```python
from build123d import *

# Parameters (mm, degrees)
SKETCH1_R           = 11
SKETCH1_R_2         = 4
SKETCH1_R_3         = 1.7
BOSS_EXTRUDE1_DEPTH = 3.5
SKETCH2_R           = 5
BOSS_EXTRUDE2_DEPTH = 10
SKETCH2_2_R         = 5
BOSS_EXTRUDE3_DEPTH = 5
SKETCH3_R           = 4
CUT_EXTRUDE1_DEPTH  = 20


with BuildPart() as part:
    # Sketch1 → Boss-Extrude1 (new body)
    with BuildSketch(Plane(origin=(0, 0, 0), x_dir=(1, 0, 0), z_dir=(0, 1, 0))):
        with Locations((-13.832754598, -13.4034603)):
            Circle(SKETCH1_R)
        with Locations((-13.832754598, -13.4034603)):
            Circle(SKETCH1_R_2, mode=Mode.SUBTRACT)
        with Locations((-19.382754598, -7.8534603)):
            Circle(SKETCH1_R_3, mode=Mode.SUBTRACT)
        with Locations((-8.282754598, -7.8534603)):
            Circle(SKETCH1_R_3, mode=Mode.SUBTRACT)
        with Locations((-8.282754598, -18.9534603)):
            Circle(SKETCH1_R_3, mode=Mode.SUBTRACT)
        with Locations((-19.382754598, -18.9534603)):
            Circle(SKETCH1_R_3, mode=Mode.SUBTRACT)
    extrude(amount=BOSS_EXTRUDE1_DEPTH)

    # Sketch2 → Boss-Extrude2 (add)
    with BuildSketch(Plane(origin=(0, 3.5, 0), x_dir=(1, 0, 0), z_dir=(0, 1, 0))):
        with Locations((-13.832754598, -13.4034603)):
            Circle(SKETCH2_R)
    extrude(amount=BOSS_EXTRUDE2_DEPTH)

    # Sketch2_2 → Boss-Extrude3 (add)
    with BuildSketch(Plane(origin=(0, 3.5, 0), x_dir=(1, 0, 0), z_dir=(0, 1, 0))):
        with Locations((-13.832754598, -13.4034603)):
            Circle(SKETCH2_2_R)
    extrude(amount=-BOSS_EXTRUDE3_DEPTH)

    # Sketch3 → Cut-Extrude1 (cut)
    with BuildSketch(Plane(origin=(0, 13.5, 0), x_dir=(1, 0, 0), z_dir=(0, 1, 0))):
        with Locations((-13.832754598, -13.4034603)):
            Circle(SKETCH3_R)
    extrude(amount=-CUT_EXTRUDE1_DEPTH, mode=Mode.SUBTRACT)


solid = part.part
```
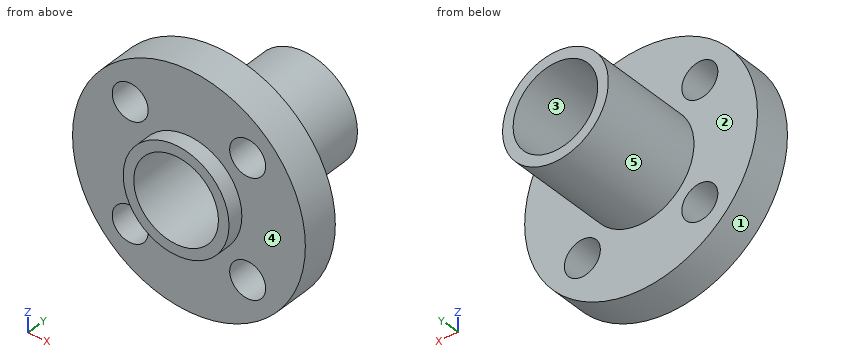
Design review of the part built by this model. Coordinates are the model's own, in mm. Face numbers are marked on the shaded views. A direction names the side the tool comes from. Give positions to 0.01 mm unless a question says otherwise; leave off trailing zeros. Loops run counter-clockwise (first coordinate to the right, second up) from the corner with the lowest first, then second, coordinate; pieces in that order, holes last. Notation, with made-up numbers: M 75,-23 L 110,-23 A12 ccw 110,-3 Z; hole C 61.5,52 d3. An arc over 180 degrees is marked long. Return JSON: item names as keys, results as strings. Group by question number.
Item 1: We need section A-A (z = 7.5). Give the boundary of the cut face in (x, y), and give its area (3 significant figures).
Item 2: Insertion check: pin 1 Ø1.5 at (y, z) = (6.5, 16) entering from -X; pin 2 Ø4.5 at (x, z) = (-8.28, 7.85) entering from -Y; pin 3 Ø8 at (y, z) = (6, 18.5) entering from -X. Each pin has a flat end and moves straight along its axis. Give the tip position at first contact, or say it passes through.
Item 3: Tool access review of the marked faces 1 and 2: name each direction out of +Z, -Z, +X, -X, +Y, -Y from which nothing blocks a thin tool from reaching the whole face with its end or side.
Item 4: Mouldability with a two-part tool opening along X and no side actions: class the marked faces 3, 4 and 5 as released by +X, released by -X, zero draft, split by the parting line, or undercut.
Item 5: We need section B-B (x = -16.5). Give the boundary of the cut face in (y, z).
Item 6: For probe 1 along Z at (x, y) = (-8.25, 0.5); probe 2 along Y at (x, z) = (-12, 18.25); probe 3 along Z at (x, y) = (-6.75, 0.25), list the stretches that pass through material, from the lowest coordinate up.
Item 7: We need section D-D (x = -8). Give the boundary of the cut face in (y, z).
Item 8: We need section C-C (z = 16). Give the boundary of the cut face in (x, y), and give its area (3 significant figures).
Output:
{
 "1": {"outline": "M -23.11,0 L -21.05,0 L -21.05,3.5 L -23.11,3.5 Z; M -17.72,0 L -9.95,0 L -9.95,3.5 L -17.72,3.5 Z; M -6.62,0 L -4.55,0 L -4.55,3.5 L -6.62,3.5 Z", "area": "41.7 mm^2"},
 "2": {"pin 1": "stops at x = -18.48", "pin 2": "stops at y = 0", "pin 3": "stops at x = -24.65"},
 "3": {"face 1": "+Y, -Y", "face 2": "+Y"},
 "4": {"face 3": "undercut", "face 4": "zero draft", "face 5": "split by the parting line"},
 "5": {"outline": "M -1.5,9.17 L 0,9.17 L 0,2.73 L 3.5,2.73 L 3.5,9.17 L 13.5,9.17 L 13.5,10.42 L -1.5,10.42 Z; M -1.5,16.38 L 13.5,16.38 L 13.5,17.63 L 3.5,17.63 L 3.5,24.08 L 0,24.08 L 0,17.63 L -1.5,17.63 Z"},
 "6": {"probe 1": "z = 3.93 to 6.15, 9.55 to 17.25, 20.65 to 22.88", "probe 2": "y = 0 to 3.5", "probe 3": "z = 4.99 to 7.12, 8.59 to 18.22, 19.69 to 21.82"},
 "7": {"outline": "M 0,4.08 L 3.5,4.08 L 3.5,6.18 L 0,6.18 Z; M 0,9.53 L 3.5,9.53 L 3.5,17.28 L 0,17.28 Z; M 0,20.63 L 3.5,20.63 L 3.5,22.73 L 0,22.73 Z"},
 "8": {"outline": "M -24.52,0 L -18.11,0 L -18.11,-1.5 L -16.88,-1.5 L -16.88,13.5 L -18.11,13.5 L -18.11,3.5 L -24.52,3.5 Z; M -10.79,-1.5 L -9.56,-1.5 L -9.56,0 L -3.14,0 L -3.14,3.5 L -9.56,3.5 L -9.56,13.5 L -10.79,13.5 Z", "area": "81.8 mm^2"}
}
